from build123d import *

# Parameters (mm, degrees)
SKETCH1_R               = 7.5
SKETCH1_R_2             = 4
BOSS_EXTRUDE1_DEPTH     = 3
CUT_EXTRUDE1_DEPTH      = 93.175105099
CUT_EXTRUDE1_DEPTH_BACK = 93.175105099
SKETCH2_R               = 1.5
SKETCH2_R_2             = 1.6
CUT_EXTRUDE3_DEPTH      = 93.175105099
CUT_EXTRUDE3_DEPTH_BACK = 93.175105099
SKETCH4_R               = 2
CUT_EXTRUDE4_DEPTH      = 10


with BuildPart() as part:
    # Sketch1 → Boss-Extrude1 (new body)
    with BuildSketch(Plane.XY):
        with BuildLine():
            Line((20, -50), (-14.482758621, -13.793103448))
            ThreePointArc((-14.482758621, -13.793103448), (-19.697630617, 3.464584837), (-8.907060148, 17.907101371))
            Line((-8.907060148, 17.907101371), (60.546469926, 52.453550686))
            ThreePointArc((60.546469926, 52.453550686), (73.60381741, 48.596501346), (70.712169365, 35.292008702))
            Line((70.712169365, 35.292008702), (20, 0))
            Line((20, 0), (60, -40))
            Line((60, -40), (60, -50))
            Line((60, -50), (20, -50))
        make_face()
        Circle(SKETCH1_R, mode=Mode.SUBTRACT)
        with Locations((65, 43.5)):
            Circle(SKETCH1_R_2, mode=Mode.SUBTRACT)
    extrude(amount=BOSS_EXTRUDE1_DEPTH)

    # Sketch2 → Cut-Extrude1 (cut, two sides: drawn at the far end of the back side and taken through both)
    with BuildSketch(Plane.XY.offset(-CUT_EXTRUDE1_DEPTH_BACK)):
        with Locations((0, 15)):
            Circle(SKETCH2_R)
        with Locations((12.990381057, -7.5)):
            Circle(SKETCH2_R)
        with Locations((-12.990381057, -7.5)):
            Circle(SKETCH2_R)
        with Locations((13.788582233, -13.788582233)):
            Circle(SKETCH2_R_2)
        with Locations((8.838834765, -8.838834765)):
            Circle(SKETCH2_R_2)
    extrude(amount=CUT_EXTRUDE1_DEPTH + CUT_EXTRUDE1_DEPTH_BACK, mode=Mode.SUBTRACT)

    # Sketch4 → Cut-Extrude3 (cut, two sides: drawn at the far end of the back side and taken through both)
    with BuildSketch(Plane.XY.offset(-CUT_EXTRUDE3_DEPTH_BACK)):
        with Locations((27, -45)):
            Circle(SKETCH4_R)
        with Locations(Location((53, -45, 0), (0, 0, 180))):
            Circle(SKETCH4_R)
    extrude(amount=CUT_EXTRUDE3_DEPTH + CUT_EXTRUDE3_DEPTH_BACK, mode=Mode.SUBTRACT)

    # Sketch5 → Cut-Extrude4 (cut)
    with BuildSketch(Plane.XY):
        with BuildLine():
            Line((60.546469926, 52.453550686), (-8.907060148, 17.907101371))
            ThreePointArc((-8.907060148, 17.907101371), (10.532302622, 17.002076387), (20, 0))
            Line((20, 0), (70.712169365, 35.292008702))
            ThreePointArc((70.712169365, 35.292008702), (73.60381741, 48.596501346), (60.546469926, 52.453550686))
        make_face()
    extrude(amount=CUT_EXTRUDE4_DEPTH, mode=Mode.SUBTRACT)


solid = part.part
Model file for the job. Use its own axes, mm. Round coordinates to 2 decimals unless told otherwise and drop trailing zeros. Loops run counter-clockwise (first coordinate to the right, second up) from the corner with the lowest first, then second, coordinate; pieces in that order, holes last. Notation, with made-up numbers: (24, 36.5) - (47, 36.5) arc R9 cw to (47, 49.5) - close; hole circle Ø8 at (-30.5, 43.25). An arc over 180 degrees is marked (long way). Write each question's results on one line, items separated by ' | '.
(1) Wall check: L1, parallel to X at y = -8, z = 0.4; L2, parallel to Y at x = 0, z = 2.35; L3, parallel to Y at x = 27, z = 1.2. Give the ranges that are in metal, low to high.
Answer below:
L1: x = -18.33 to -14.4, -11.58 to 7.48, 10.2 to 11.58, 14.4 to 28 | L2: y = -29 to -7.5, 7.5 to 13.5, 16.5 to 20 | L3: y = -50 to -47, -43 to -7
(2) Pin check, flat tips, straight feed: pin 1 (3.5 mm diameter, centred on x = 12.99, y = -7.5, fed in from +Z); pin 2 (1.5 mm diameter, centred on x = 22.5, z = 2, fed in from +Y); pin 3 (1 mm diameter, centred on x = 26.5, z = 0.5, fed in from +Y). Stop position of each tip, or through.
Answer below:
pin 1: stops at z = 3 | pin 2: stops at y = -1.75 | pin 3: stops at y = -6
(3) Saw through at D-D, the plane z = 1.7. Count the separate pieces of the cut face and the enclosed holes in it, then the cut area to 3 significant figures.
Answer below:
separate pieces: 1 | enclosed holes: 8 | area: 2,740 mm^2
(4) Saw through at B-B, the plane y = -45. List the corners of the cut face in (x, z).
Answer below:
outline: (15.24, 0) - (25, 0) - (25, 3) - (15.24, 3) - close; (29, 0) - (51, 0) - (51, 3) - (29, 3) - close; (55, 0) - (60, 0) - (60, 3) - (55, 3) - close
(5) Saw through at C-C, the plane y = 5.5. List the corners of the cut face in (x, z).
Answer below:
outline: (-19.23, 0) - (-5.1, 0) - (-5.1, 3) - (-19.23, 3) - close; (5.1, 0) - (19.23, 0) - (19.23, 3) - (5.1, 3) - close
(6) Mould opens along X. For faces 1 (the flat face through (40, -50, 1)), 2 (the flat face through (60, -45, 1)), 3 (the cylindrical face through (12.19, -13.72, 1.48)) say: released by +X, released by -X, zero draft, split by the parting line, or undercut.
Answer below:
face 1: zero draft | face 2: released by +X | face 3: undercut
(7) Saw through at A-A, the plane x = 53. List the corners of the cut face in (y, z), then the cut area to 3 significant figures.
Answer below:
outline: (-50, 0) - (-47, 0) - (-47, 3) - (-50, 3) - close; (-43, 0) - (-33, 0) - (-33, 3) - (-43, 3) - close | area: 39.0 mm^2
